Check sheet for the drawn part. Datum: minimum x, y, z corner. Units: mm. Give positions to 0.01 mm unless a question says otherwise; leave off trailing zeros. Write each loop counter-clockwise with the first axis right and the second up, starting at its lowest first coordinate (ties: lowest second). Pieces come first, ordered by that corner, then holes. Notation, with made-up numbers: (88.25, -17.75) - (105.25, -17.75) arc R24 ccw to (105.25, 3.25) - close; hole circle Ø9 at (88.25, 60). An arc over 180 degrees is marked (long way). Answer as a JSON object with one key per item and string values. Group by question number.
Item 1: Scan lines: line 1 along X through (y, z) = (2.4, 11); line 2 along X through (y, z) = (1.9, 19); line 3 along Z through (x, y) = (11.25, 2.1). Record each from-to range of solid material in increasing order. Write a range as [from, to].
Item 2: Sectioned sample at C-C, the plane y = 0.65. Record the boundary of the cut face in (x, z).
Item 3: Sectioned sample at D-D, the plane z = 11. Record the boundary of the cut face in (x, y) (3 decimals).
Item 4: Draft check along X on the marked faces 1, 2, 3 and 4. Enter one of: +X half, -X half, draft (parallel to the pull), parting line (faces both ways), or undercut.
Item 5: Sectioned sample at A-A, the plane z = 3. Record the boundary of the cut face in (x, y) (3 decimals), and give its area (3 significant figures).
Item 6: Sectioned sample at B-B, the plane x = 19. Record the boundary of the cut face in (y, z) (3 decimals).
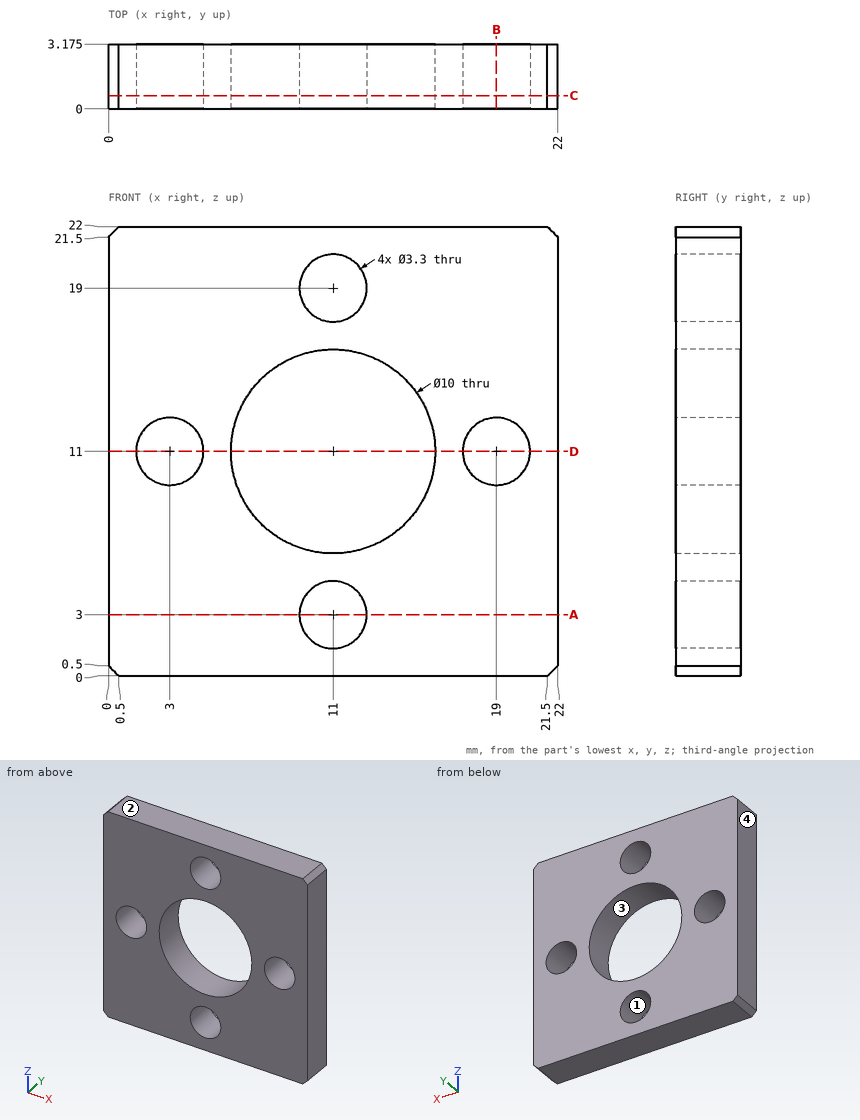
Geometry check:
{
 "1": {"line 1": "[0, 1.35], [4.65, 6], [16, 17.35], [20.65, 22]", "line 2": "[0, 9.35], [12.65, 22]", "line 3": "[0, 1.37], [4.63, 6.01], [15.99, 17.37], [20.63, 22]"},
 "2": {"outline": "(0, 0.5) - (0.5, 0) - (21.5, 0) - (22, 0.5) - (22, 21.5) - (21.5, 22) - (0.5, 22) - (0, 21.5) - close; hole circle Ø3.3 at (3, 11); hole circle Ø10 at (11, 11); hole circle Ø3.3 at (11, 3); hole circle Ø3.3 at (11, 19); hole circle Ø3.3 at (19, 11)"},
 "3": {"outline": "(0, 0) - (1.35, 0) - (1.35, 3.175) - (0, 3.175) - close; (4.65, 0) - (6, 0) - (6, 3.175) - (4.65, 3.175) - close; (16, 0) - (17.35, 0) - (17.35, 3.175) - (16, 3.175) - close; (20.65, 0) - (22, 0) - (22, 3.175) - (20.65, 3.175) - close"},
 "4": {"face 1": "undercut", "face 2": "draft", "face 3": "undercut", "face 4": "-X half"},
 "5": {"outline": "(0, 0) - (9.35, 0) - (9.35, 3.175) - (0, 3.175) - close; (12.65, 0) - (22, 0) - (22, 3.175) - (12.65, 3.175) - close", "area": "59.4 mm^2"},
 "6": {"outline": "(0, 0) - (3.175, 0) - (3.175, 9.35) - (0, 9.35) - close; (0, 12.65) - (3.175, 12.65) - (3.175, 22) - (0, 22) - close"}
}
